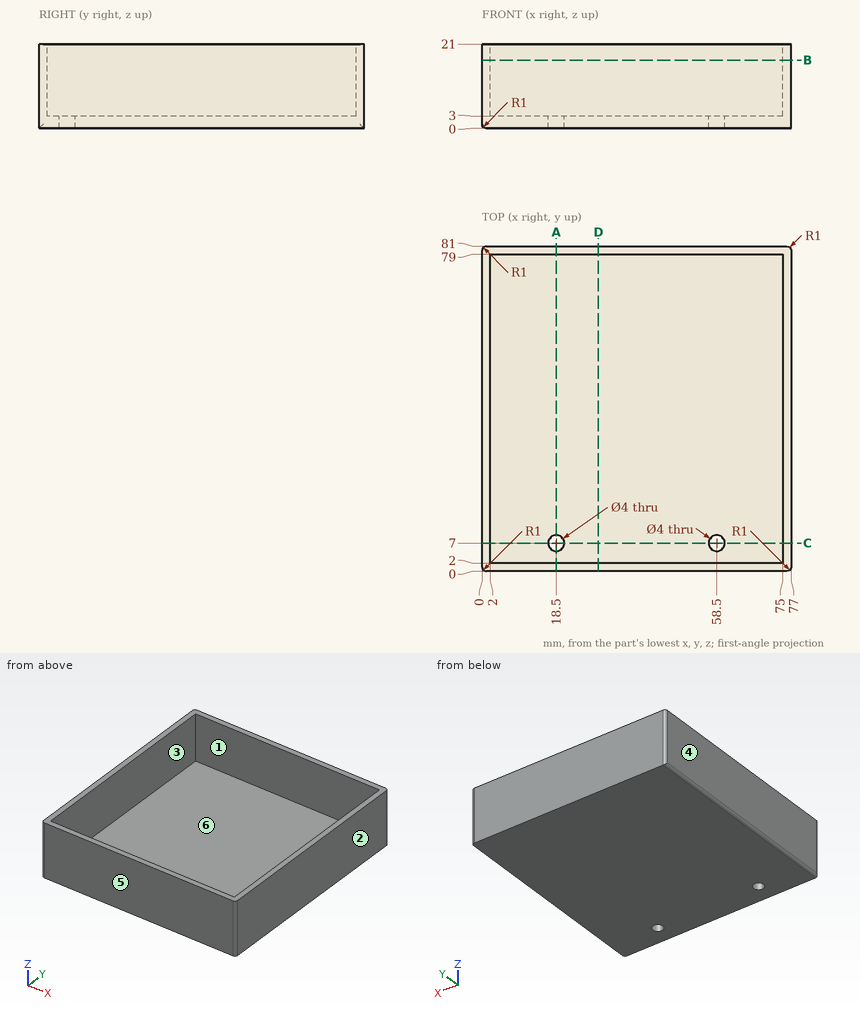
Geometry check sheet. Reference: drawing and pictorial views, mm from the part's lowest x, y, z. A direction names the side the tool comes from. Coordinates: 2 decimals unless noted, no trailing zeros. Order: outer loops, then holes, each group sorted by start corner. A loop starts at its lowest first (then second) coordinate and runs counter-clockwise, first axis right, second up.
1. Scan lines: line 1 (X direction, y = 7, z = 1.3); line 2 (Y direction, x = 19, z = 17.5); line 3 (X direction, y = 21.5, z = 5.75). Record each from-to range of solid material in increasing order.
Results found:
line 1: x = 0 to 16.5, 20.5 to 56.5, 60.5 to 77
line 2: y = 0 to 2, 79 to 81
line 3: x = 0 to 2, 75 to 77
2. Go/stop test with flat-tipped pins: pin 1 Ø2.5 at (x, y) = (18.5, 7) entering from -Z; pin 2 Ø2 at (x, y) = (10, 69) entering from +Z. Record where each tip stops, or that it passes through.
Results found:
pin 1: passes through
pin 2: stops at z = 3
3. Sectioned sample at B-B, the plane z = 17. Record the cut outline in (x, y), and give its area (3 significant figures).
Results found:
outline: (0, 1) arc R1 ccw to (1, 0) - (76, 0) arc R1 ccw to (77, 1) - (77, 80) arc R1 ccw to (76, 81) - (1, 81) arc R1 ccw to (0, 80) - close; hole (2, 2) - (75, 2) - (75, 79) - (2, 79) - close
area: 615 mm2
4. Sectioned sample at A-A, the plane x = 18.5. Record the cut outline in (y, z).
Results found:
outline: (0, 0) - (5, 0) - (5, 3) - (2, 3) - (2, 21) - (0, 21) - close; (9, 0) - (81, 0) - (81, 21) - (79, 21) - (79, 3) - (9, 3) - close
5. Sectioned sample at C-C, the plane y = 7. Record the cut outline in (x, z), and give its area (3 significant figures).
Results found:
outline: (0, 1) arc R1 ccw to (1, 0) - (16.5, 0) - (16.5, 3) - (2, 3) - (2, 21) - (0, 21) - close; (20.5, 0) - (56.5, 0) - (56.5, 3) - (20.5, 3) - close; (60.5, 0) - (77, 0) - (77, 21) - (75, 21) - (75, 3) - (60.5, 3) - close
area: 279 mm2
6. Release check for a two-part mould opening along X. For the marked faces 3, 4, 5 and 6 record: +X half, -X half, draft (parallel to the pull), parting line (faces both ways), or undercut.
Results found:
face 3: undercut
face 4: -X half
face 5: draft
face 6: undercut
7. Set-up check for the marked faces 1 and 2: record each of +Z, -Z, +X, -X, +Y, -Y from which the full face is reachable in a straight line by a thin tool's end or side.
Results found:
face 1: +Z
face 2: +Z, -Z, +X, +Y, -Y
8. Sectioned sample at D-D, the plane x = 29. Record the cut outline in (y, z), and give its area (3 significant figures).
Results found:
outline: (0, 0) - (81, 0) - (81, 21) - (79, 21) - (79, 3) - (2, 3) - (2, 21) - (0, 21) - close
area: 315 mm2
